Geometry check sheet. Reference: the model listing, model coordinates, mm. Round coordinates to 2 decimals unless told otherwise and drop trailing zeros. Loops run counter-clockwise (first coordinate to the right, second up) from the corner with the lowest first, then second, coordinate; pieces in that order, holes last. Notation, with made-up numbers: (-14.5, 41) -> (-5.5, 41) arc R20 cw to (-5.5, 51) -> close; hole circle Ø7 at (85.25, -7.5). An arc over 180 degrees is marked (long way). Use one line per item in the form item = value.
from build123d import *

# Parameters (mm, degrees)
F0_R        = 15
F0_R_2      = 12.5
F2_DEPTH    = 2
F3_DEPTH    = 2
F5_T2_ANGLE = 356.0811167668
F5_T4_ANGLE = 356.0811167668


# Not quite as in the source:
# - a fillet or chamfer that OpenCascade refuses, or shapes differently, is made with other operations: its cross-section is extruded or revolved along the edge and cut away or added


with BuildPart() as f2:
    # F0 (on Front) → F2 (new body, symmetric)
    with BuildSketch(Plane.XZ):
        Circle(F0_R)
        Circle(F0_R_2, mode=Mode.SUBTRACT)
    extrude(amount=F2_DEPTH, both=True)


with BuildPart() as f3:
    # F1 (on Front) → F3 (new body, symmetric)
    with BuildSketch(Plane.XZ):
        Polygon((14.1155660557, -0.6062071938), (14.654473997, -0.9977467319), (15.3206008461, -0.9977467319), (15.8595087875, -0.6062071938), (16.0653533043, 0.0273170867), (15.8595087875, 0.6608413673), (15.4207458886, 1.032837417), (14.98814394, 1.032837417), (14.4956499742, 1.032837417), (14.1155660557, 0.6608413673), (13.9097215389, 0.0273170867), align=None)
    extrude(amount=F3_DEPTH, both=True)


with BuildPart() as f3b:
    # F1 (on Front) → F3, piece 2 (new body, symmetric)
    with BuildSketch(Plane.XZ):
        Polygon((14.5303690806, 1.108682598), (14.9253355339, 1.0592561448), (14.7739350796, 1.3965530088), (14.6046532318, 1.5607766109), (14.1262672842, 1.6433858545), (14.2477648333, 1.2773335911), align=None)
    extrude(amount=F3_DEPTH, both=True)


with BuildPart() as f3c:
    # F1 (on Front) → F3, piece 3 (new body, symmetric)
    with BuildSketch(Plane.XZ):
        Polygon((15.1731697154, 1.4260609763), (14.9909034371, 1.0592561448), (15.3603749383, 1.0987263252), (15.5725924471, 1.2016314485), (15.8138373742, 1.622913168), (15.4283061543, 1.6339400652), align=None)
    extrude(amount=F3_DEPTH, both=True)


with BuildPart() as f2_1:
    add(f2.part)

    # F4: cut F3, F3c, F3b
    add(f3.part, mode=Mode.SUBTRACT)
    add(f3c.part, mode=Mode.SUBTRACT)
    add(f3b.part, mode=Mode.SUBTRACT)

    # F5: fillet of radius 0.2 on 2 edges, made by hand

    # F5_s1 → F5_t2 (revolve, cut)
    with BuildSketch(Plane(origin=(0, 0, 0), x_dir=(0, 1, 0), z_dir=(0.0353637111, 0, -0.9993745084))):
        with BuildLine():
            ThreePointArc((-1.8, 15), (-1.9414213562, 14.9414213562), (-2, 14.8))
            Line((-2, 14.8), (-2, 15))
            Line((-2, 15), (-1.8, 15))
        make_face()
    revolve(axis=Axis((0, -2, 0), (0, -1, 0)), revolution_arc=F5_T2_ANGLE, mode=Mode.SUBTRACT)

    # F5_s3 → F5_t4 (revolve, cut)
    with BuildSketch(Plane(origin=(0, 0, 0), x_dir=(0, 1, 0), z_dir=(0.0353637111, 0, -0.9993745084))):
        with BuildLine():
            ThreePointArc((1.8, 15), (1.9414213562, 14.9414213562), (2, 14.8))
            Line((2, 14.8), (2, 15))
            Line((2, 15), (1.8, 15))
        make_face()
    revolve(axis=Axis((0, 2, 0), (0, -1, 0)), revolution_arc=F5_T4_ANGLE, mode=Mode.SUBTRACT)


solid = f2_1.part
1. Material ranges on line 1 along Z through (x, y) = (0, -0.25); line 2 along X through (y, z) = (0, 0.5); line 3 along X through (y, z) = (-0.2, 6), recorded low to high.
Return value:
line_1 = -15 to -12.5, 12.5 to 15
line_2 = -14.99 to -12.49, 12.49 to 14.06
line_3 = -13.75 to -10.97, 10.97 to 13.75
2. Gauge pin test, flat end, axial feed: pin 1 (1.5 mm diameter, centred on x = -7, y = 1.5, fed in from +Z). Record the tip position at first contact, or that the pin passes through.
Return value:
pin_1 = 13.64
3. Section check A-A (x = 0). Record the boundary of the cut face in (y, z).
Return value:
outline = (-2, -14.8) arc R0.2 ccw to (-1.8, -15) -> (1.8, -15) arc R0.2 ccw to (2, -14.8) -> (2, -12.5) -> (-2, -12.5) -> close; (-2, 12.5) -> (2, 12.5) -> (2, 14.8) arc R0.2 ccw to (1.8, 15) -> (-1.8, 15) arc R0.2 ccw to (-2, 14.8) -> close
4. Section check B-B (y = -0.25). Record the boundary of the cut face in (x, z), then the cut area to 3 significant figures.
Return value:
outline = (13.91, 0.03) -> (14.12, 0.66) -> (14.5, 1.03) -> (14.96, 1.03) arc R15 ccw (long way) to (14.97, -1) -> (14.65, -1) -> (14.12, -0.61) -> close; hole circle Ø25 at (0, 0); hole (14.13, 1.64) -> (14.25, 1.28) -> (14.53, 1.11) -> (14.93, 1.06) -> (14.77, 1.4) -> (14.6, 1.56) -> close
area = 214 mm2
5. Mould release check, pull along X, two halves, no side actions. Record for faces 1 (the cylindrical face through (11.923, 0.028, 3.755)), 2 (the cylindrical face through (-14.987, -0.025, 0.628)), 3 (the flat face through (-9, -2, 9)): released by +X, released by -X, zero draft, split by the parting line, or undercut.
Return value:
face_1 = undercut
face_2 = split by the parting line
face_3 = zero draft
